Geometry: final body of the model. Coordinates: model frame, mm. Give positions to 0.01 mm unless a question says otherwise; leave off trailing zeros. Write each loop counter-clockwise with the first axis right and the second up, starting at its lowest first coordinate (ties: lowest second). Pieces come first, ordered by that corner, then holes.
Q1. Section A-A (x = 0). Return the cut outline in (y, z), plus the area to 3 significant figures.
Q2. Pin query (flat end, axial travel): pin 1 Ø10 at (y, z) = (7.5, 120.5) entering from -X; pin 2 Ø12 at (x, z) = (6.5, 59) entering from +Y; pin 3 Ø6.5 at (x, z) = (1.5, 175) entering from +Y. Return the tip coordinate at first contact, or that it passes through.
Q3. Section C-C (z = 10). Return the cut outline in (x, y), plus the area to 3 significant figures.
Q4. Section D-D (z = 148.5). Return the cut outline in (x, y).
Q5. Line query: line 1 (Z direction, x = 0, y = -5.5); line 2 (X direction, y = 0.25, z = 10); line 3 (Z direction, x = 0.75, y = 1). Output: solid intervals per line, ascending.
Q6. Section B-B (y = -6). Return the cut outline in (x, z), plus the area to 3 significant figures.
from build123d import *

# Parameters (mm, degrees)
SKETCH1_R               = 10
BOSS_EXTRUDE1_DEPTH     = 180
CUT_EXTRUDE1_DEPTH      = 181.554700853
CUT_EXTRUDE1_DEPTH_BACK = 181.554700853
SKETCH2_R               = 4
CUT_EXTRUDE2_START      = -10
CUT_EXTRUDE2_DEPTH      = 10


with BuildPart() as part:
    # Sketch1 → Boss-Extrude1 (new body)
    with BuildSketch(Plane.XY):
        with Locations(Location((0, 0, 0), (0, 0, 180))):
            Circle(SKETCH1_R)
    extrude(amount=BOSS_EXTRUDE1_DEPTH)

    # Sketch2 → Cut-Extrude1 (cut, two sides: drawn at the far end of the back side and taken through both)
    with BuildSketch(Plane(origin=(0, 0, 0), x_dir=(1, 0, 0), z_dir=(0, 1, 0)).offset(-CUT_EXTRUDE1_DEPTH_BACK)):
        with Locations(Location((0, -10, 0), (0, 0, 270))):
            Circle(SKETCH2_R)
    extrude(amount=CUT_EXTRUDE1_DEPTH + CUT_EXTRUDE1_DEPTH_BACK, mode=Mode.SUBTRACT)

    # Sketch3 → Cut-Extrude2 (cut)
    with BuildSketch(Plane.XY.offset(180).offset(CUT_EXTRUDE2_START)):
        with BuildLine():
            Line((-4.161531139, 9.092945539), (4.161531139, 9.092945539))
            ThreePointArc((4.161531139, 9.092945539), (0, 10), (-4.161531139, 9.092945539))
        make_face()
    extrude(amount=CUT_EXTRUDE2_DEPTH, mode=Mode.SUBTRACT)


solid = part.part
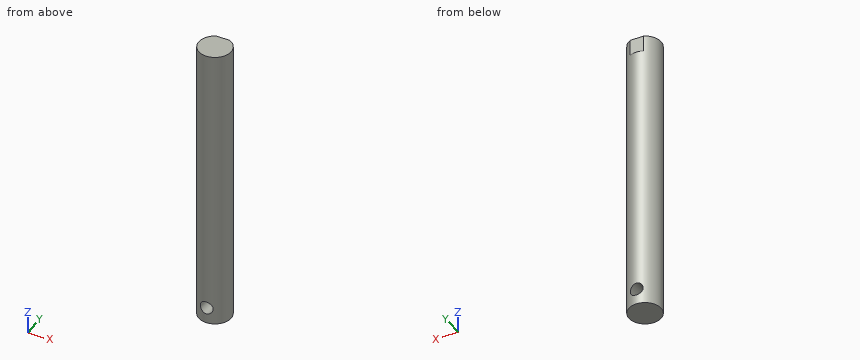
Computed:
1. outline: (-10, 0) - (10, 0) - (10, 6) - (-10, 6) - close; (-10, 14) - (10, 14) - (10, 170) - (9.09, 170) - (9.09, 180) - (-10, 180) - close
1. area: 3,430 mm2
2. pin 1: stops at x = -9.68
2. pin 2: stops at y = 9.99
2. pin 3: stops at y = 9.09
3. outline: (-4, -9.17) - (-4, 9.17) arc R10 ccw to start; (4, -9.17) arc R10 ccw to (4, 9.17) - close
3. area: 159 mm2
4. outline: circle Ø20 at (0, 0)
5. line 1: z = 0 to 6, 14 to 180
5. line 2: x = -10 to -4, 4 to 10
5. line 3: z = 0 to 6.07, 13.93 to 180
6. outline: (-8, 0) - (8, 0) - (8, 180) - (-8, 180) - close; hole circle Ø8 at (0, 10)
6. area: 2,830 mm2
